```python
from build123d import *

# Parameters (mm, degrees)
SKETCH1_R           = 42.5
BOSS_EXTRUDE1_DEPTH = 23
SKETCH2_R           = 7.5
CUT_EXTRUDE1_DEPTH  = 65.354487023
SKETCH3_R           = 1.721944662
CUT_EXTRUDE2_DEPTH  = 21.068692
CIRPATTERN1_START   = 1.93130801
CIRPATTERN1_DEPTH   = 21.06869199


# Read off the part's stored shape, not the designer's step: CirPattern1
with BuildPart() as part:
    # Sketch1 → Boss-Extrude1 (new body)
    with BuildSketch(Plane(origin=(0, 0, 0), x_dir=(1, 0, 0), z_dir=(0, 1, 0))):
        with Locations(Location((0, 0, 0), (0, 0, 270))):
            Circle(SKETCH1_R)
    extrude(amount=BOSS_EXTRUDE1_DEPTH)

    # Sketch2 → Cut-Extrude1 (cut, through all)
    with BuildSketch(Plane(origin=(0, 0, 0), x_dir=(1, 0, 0), z_dir=(0, 1, 0))):
        with Locations(Location((0, 0, 0), (0, 0, 270))):
            Circle(SKETCH2_R)
    extrude(amount=CUT_EXTRUDE1_DEPTH, mode=Mode.SUBTRACT)

    # Sketch3 → Cut-Extrude2 (cut)
    with BuildSketch(Plane(origin=(0, 23, 0), x_dir=(1, 0, 0), z_dir=(0, 1, 0))):
        with Locations((-6.236582965, 0)):
            Circle(SKETCH3_R)
    extrude(amount=-CUT_EXTRUDE2_DEPTH, mode=Mode.SUBTRACT)

    # CirPattern1 outline → CirPattern1 (cut)
    with BuildSketch(Plane(origin=(0, 0, 0), x_dir=(1, 0, 0), z_dir=(0, 1, 0)).offset(CIRPATTERN1_START)):
        with BuildLine():
            ThreePointArc((-2.588058657, -7.039314767), (-3.75, -6.495190528), (-4.802196085, -5.760981927))
            ThreePointArc((-4.802196085, -5.760981927), (-3.979263814, -6.892287102), (-2.588058657, -7.039314767))
        make_face()
        with BuildLine():
            ThreePointArc((-2.588058657, 7.039314767), (-3.979263814, 6.892287102), (-4.802196085, 5.760981927))
            ThreePointArc((-4.802196085, 5.760981927), (-3.75, 6.495190528), (-2.588058657, 7.039314767))
        make_face()
        with BuildLine():
            ThreePointArc((4.802196085, -5.760981927), (3.75, -6.495190528), (2.588058657, -7.039314767))
            ThreePointArc((2.588058657, -7.039314767), (3.979263814, -6.892287102), (4.802196085, -5.760981927))
        make_face()
        with BuildLine():
            ThreePointArc((4.802196085, 5.760981927), (3.979263814, 6.892287102), (2.588058657, 7.039314767))
            ThreePointArc((2.588058657, 7.039314767), (3.75, 6.495190528), (4.802196085, 5.760981927))
        make_face()
        with BuildLine():
            ThreePointArc((7.390254742, 1.27833284), (7.5, 0), (7.390254742, -1.27833284))
            ThreePointArc((7.390254742, -1.27833284), (7.958527627, 0), (7.390254742, 1.27833284))
        make_face()
    extrude(amount=CIRPATTERN1_DEPTH, mode=Mode.SUBTRACT)


solid = part.part
```
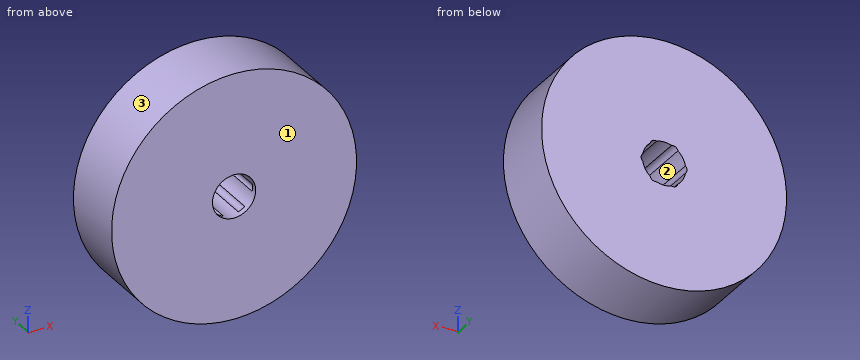
Read the model definition and answer for the solid it produces. Units are mm, in the model's axes. Face numbers are marked on the shaded views. Round coordinates to 2 decimals unless told otherwise and drop trailing zeros. Loops run counter-clockwise (first coordinate to the right, second up) from the corner with the lowest first, then second, coordinate; pieces in that order, holes last. Notation, with made-up numbers: (77, -33.5) -> (88, -33.5) arc R14 cw to (88, -17.5) -> close; hole circle Ø4 at (78, 8.25). An arc over 180 degrees is marked (long way). One line per item, written item: value.
1) A cutting plane is placed at A-A (z = 0). Determine the outline of the cut face in (x, y).
Answer list:
outline: (-42.5, 0) -> (-7.5, 0) -> (-7.5, 1.93) -> (-7.96, 1.93) -> (-7.96, 23) -> (-42.5, 23) -> close; (7.5, 0) -> (42.5, 0) -> (42.5, 23) -> (7.96, 23) -> (7.96, 1.93) -> (7.5, 1.93) -> close
2) Flat-ended cylindrical pins translate along their axes: P1, Ø4, axis at y = 16.5, z = 12, coming from the -X side; P2, Ø1.5, axis at x = -26.5, y = 12, coming from the +Z side; P3, Ø4, axis at y = 20.5, z = 5.5, coming from the +X side; P4, Ø13.5, axis at x = 0, z = 0, coming from the +Y side. Find the tip coordinate at first contact, or state that the pin passes through.
Answer list:
P1: stops at x = -41.31
P2: stops at z = 33.81
P3: stops at x = 42.36
P4: passes through
3) A cutting plane is placed at C-C (y = 3.5). Determine the outline of the cut face in (x, z).
Answer list:
outline: circle Ø85 at (0, 0); hole (-7.39, -1.28) arc R7.5 ccw to (-4.8, -5.76) arc R1.72 ccw to (-2.59, -7.04) arc R7.5 ccw to (2.59, -7.04) arc R1.72 ccw to (4.8, -5.76) arc R7.5 ccw to (7.39, -1.28) arc R1.72 ccw to (7.39, 1.28) arc R7.5 ccw to (4.8, 5.76) arc R1.72 ccw to (2.59, 7.04) arc R7.5 ccw to (-2.59, 7.04) arc R1.72 ccw to (-4.8, 5.76) arc R7.5 ccw to (-7.39, 1.28) arc R1.72 ccw to start
4) A cutting plane is placed at D-D (x = -18). Determine the outline of the cut face in (y, z).
Answer list:
outline: (0, -38.5) -> (23, -38.5) -> (23, 38.5) -> (0, 38.5) -> close
5) The mould has two halves that part along X. Classify the marked faces 1, 2 and 3: pulls with the +X half, pulls with the -X half, needs draft (parallel to the pull), parting line crosses it, or undercut.
Answer list:
face 1: needs draft
face 2: undercut
face 3: parting line crosses it
6) Consider L1, parallel to X at y = 6.25, z = -5; L2, parallel to X at y = 17.5, z = 2. Determine where each line is inside the solid, lowest interval first. Write a range as [from, to].
Answer list:
L1: x = [-42.2, -5.59], [5.59, 42.2]
L2: x = [-42.45, -7.23], [7.23, 42.45]
7) A cutting plane is placed at B-B (x = 0). Determine the outline of the cut face in (y, z), and give its area (3 significant figures).
Answer list:
outline: (0, -42.5) -> (23, -42.5) -> (23, -7.5) -> (0, -7.5) -> close; (0, 7.5) -> (23, 7.5) -> (23, 42.5) -> (0, 42.5) -> close
area: 1,610 mm²
